Autodesk Inventor part; units mm, degrees
ref_plane "Work Plane2" through (0, 130.175, -69.85) normal (0, 1, 0) x (1, 0, 0)
ref_plane "YZ Plane" through (0, 0, 0) normal (1, 0, 0) x (0, 1, 0)
ref_plane "XZ Plane" through (0, 0, 0) normal (0, 1, 0) x (-1, 0, 0)
ref_plane "Work Plane2" through (0, 130.175, -69.85) normal (0, 1, 0) x (1, 0, 0)
sketch "Sketch3" plane through (0, 130.175, -69.85) normal (0, 1, 0) x (1, 0, 0)
  line L0 (466.5934, -88.9) -> (346.2066, -88.9)
  arc A0 (343.457, -87.3125) -> (346.2066, -88.9) centre (346.2066, -85.725) ccw
  line L1 (334.2915, -71.4375) -> (343.457, -87.3125)
  line L2 (453.2877, 2.1413) -> (445.3167, 25.2907)
  arc A1 (445.3167, 25.2907) -> (442.3147, 27.432) centre (442.3147, 24.257) ccw
  line L3 (370.4853, 27.432) -> (442.3147, 27.432)
  arc A2 (370.4853, 27.432) -> (367.4833, 25.2907) centre (370.4853, 24.257) ccw
  line L4 (367.4833, 25.2907) -> (359.5123, 2.1413)
  arc A3 (356.5103, 0) -> (359.5123, 2.1413) centre (356.5103, 3.175) ccw
  line L5 (355.6, 0) -> (356.5103, 0)
  line L6 (355.6, 0) -> (0, 0)
  line L7 (0, 0) -> (0, -69.85)
  line L8 (0, -69.85) -> (330.2, -69.85)
  line L9 (330.2, -69.85) -> (331.5419, -69.85)
  arc A4 (334.2915, -71.4375) -> (331.5419, -69.85) centre (331.5419, -73.025) ccw
  line L10 (334.2915, -71.4375) -> (343.457, -87.3125)
  arc A5 (343.457, -87.3125) -> (346.2066, -88.9) centre (346.2066, -85.725) ccw
  line L11 (466.5934, -88.9) -> (346.2066, -88.9)
  arc A6 (466.5934, -88.9) -> (469.343, -87.3125) centre (466.5934, -85.725) ccw
  line L12 (469.343, -87.3125) -> (478.5085, -71.4375)
  arc A7 (481.2581, -69.85) -> (478.5085, -71.4375) centre (481.2581, -73.025) ccw
  line L13 (481.2581, -69.85) -> (482.6, -69.85)
  line L14 (482.6, -69.85) -> (812.8, -69.85)
  line L15 (812.8, -69.85) -> (812.8, 0)
  line L16 (812.8, 0) -> (457.2, 0)
  line L17 (456.2897, 0) -> (457.2, 0)
  arc A8 (453.2877, 2.1413) -> (456.2897, 0) centre (456.2897, 3.175) ccw
  circle A9 centre (619.3642, -13.4813) radius 2.667
  circle A10 centre (193.4358, -13.4813) radius 2.667
  circle A11 centre (193.4358, -60.1787) radius 2.667
  arc A12 (666.4551, -57.5409) -> (666.4551, -62.8165) centre (666.0616, -60.1787) ccw
  arc A13 (666.4551, -62.8165) -> (666.4551, -57.5409) centre (666.8486, -60.1787) ccw
  arc A14 (146.3449, -16.1191) -> (146.3449, -10.8435) centre (146.7384, -13.4813) ccw
  arc A15 (146.3449, -10.8435) -> (146.3449, -16.1191) centre (145.9514, -13.4813) ccw
  arc A16 (146.3449, -62.8165) -> (146.3449, -57.5409) centre (146.7384, -60.1787) ccw
  arc A17 (146.3449, -57.5409) -> (146.3449, -62.8165) centre (145.9514, -60.1787) ccw
  arc A18 (666.4551, -10.8435) -> (666.4551, -16.1191) centre (666.0616, -13.4813) ccw
  arc A19 (666.4551, -16.1191) -> (666.4551, -10.8435) centre (666.8486, -13.4813) ccw
  circle A20 centre (170.0871, -36.83) radius 9.525
  circle A21 centre (619.3642, -60.1787) radius 2.667
  circle A22 centre (642.7129, -36.83) radius 9.525
  circle A23 centre (122.6027, -36.83) radius 9.525
  circle A24 centre (99.254, -60.1787) radius 2.667
  circle A25 centre (99.254, -13.4813) radius 2.667
  circle A26 centre (713.546, -13.4813) radius 2.667
  circle A27 centre (713.546, -60.1787) radius 2.667
  circle A28 centre (690.1973, -36.83) radius 9.525
  circle A29 centre (461.9625, -82.7405) radius 3.4036
  circle A30 centre (350.8375, -82.7405) radius 3.4036
  circle A31 centre (711.2, -3.175) radius 1.27
  circle A32 centre (711.2, -66.675) radius 1.27
  circle A33 centre (762, -66.675) radius 1.27
  circle A34 centre (762, -3.175) radius 1.27
  circle A35 centre (50.8, -66.675) radius 1.27
  circle A36 centre (50.8, -3.175) radius 1.27
  circle A37 centre (101.6, -3.175) radius 1.27
  circle A38 centre (101.6, -66.675) radius 1.27
  circle A39 centre (806.45, -30.353) radius 3.3528
  circle A40 centre (6.35, -30.353) radius 3.3528
  circle A41 centre (787.4, -8.128) radius 3.3528
  circle A42 centre (685.8, -8.128) radius 3.3528
  circle A43 centre (584.2, -8.128) radius 3.3528
  circle A44 centre (533.4, -8.128) radius 3.3528
  circle A45 centre (482.6, -8.128) radius 3.3528
  circle A46 centre (25.4, -8.128) radius 3.3528
  circle A47 centre (127, -8.128) radius 3.3528
  circle A48 centre (228.6, -8.128) radius 3.3528
  circle A49 centre (279.4, -8.128) radius 3.3528
  circle A50 centre (330.2, -8.128) radius 3.3528
  circle A51 centre (450.8881, -70.8889) radius 2.032
  circle A52 centre (361.9119, -70.8889) radius 2.032
  circle A53 centre (367.7539, -70.8889) radius 2.54
  circle A54 centre (445.0461, -70.8889) radius 2.54
  circle A55 centre (368.808, 18.0035) radius 2.032
  circle A56 centre (443.992, 18.0035) radius 2.032
  circle A57 centre (374.65, 18.0035) radius 2.54
  circle A58 centre (438.15, 18.0035) radius 2.54
  circle A59 centre (367.6757, 1.016) radius 4.7625
  circle A60 centre (367.6757, -49.784) radius 4.7625
  circle A61 centre (445.1243, -49.784) radius 4.7625
  circle A62 centre (445.1243, 1.016) radius 4.7625
  circle A63 centre (367.6757, -24.384) radius 4.7625
  circle A64 centre (445.1243, -24.384) radius 4.7625
  circle A65 centre (406.4, -11.8872) radius 11.1125
  circle A66 centre (641.35, -55.118) radius 3.3528
  circle A67 centre (546.1, -55.118) radius 3.3528
  circle A68 centre (266.7, -55.118) radius 3.3528
  circle A69 centre (171.45, -55.118) radius 3.3528
  circle A70 centre (513.9255, -52.3027) radius 3.3528
  circle A71 centre (298.8745, -52.3027) radius 3.3528
  circle A72 centre (628.9477, -50.8) radius 4.826
  circle A73 centre (601.4385, -50.8) radius 4.826
  circle A74 centre (568.9249, -50.8) radius 4.826
  circle A75 centre (243.8751, -50.8) radius 4.826
  circle A76 centre (211.3615, -50.8) radius 4.826
  circle A77 centre (183.8523, -50.8) radius 4.826
  circle A78 centre (678.9442, -49.022) radius 4.826
  circle A79 centre (701.4504, -49.022) radius 4.826
  circle A80 centre (726.4609, -49.022) radius 4.826
  circle A81 centre (133.8558, -49.022) radius 4.826
  circle A82 centre (111.3496, -49.022) radius 4.826
  circle A83 centre (86.3391, -49.022) radius 4.826
  circle A84 centre (406.4, -52.578) radius 14.2875
  line L18 (826.5143, 100.4197) -> (706.1275, 100.4197)
  line L19 (813.2086, 191.4611) -> (805.2376, 214.6104)
  arc A85 (805.2376, 214.6104) -> (802.2356, 216.7517) centre (802.2356, 213.5767) ccw
  line L20 (730.4062, 216.7517) -> (802.2356, 216.7517)
  arc A86 (730.4062, 216.7517) -> (727.4042, 214.6104) centre (730.4062, 213.5767) ccw
  line L21 (727.4042, 214.6104) -> (719.4332, 191.4611)
  arc A87 (716.4312, 189.3197) -> (719.4332, 191.4611) centre (716.4312, 192.4947) ccw
  line L22 (715.5209, 189.3197) -> (716.4312, 189.3197)
  line L23 (826.5143, 100.4197) -> (706.1275, 100.4197)
  arc A88 (826.5143, 100.4197) -> (829.2639, 102.0072) centre (826.5143, 103.5947) ccw
  line L24 (816.2106, 189.3197) -> (817.1209, 189.3197)
  arc A89 (813.2086, 191.4611) -> (816.2106, 189.3197) centre (816.2106, 192.4947) ccw
  circle A90 centre (821.8834, 106.5792) radius 3.4036
  circle A91 centre (710.7584, 106.5792) radius 3.4036
  circle A92 centre (810.809, 118.4309) radius 2.032
  circle A93 centre (721.8328, 118.4309) radius 2.032
  circle A94 centre (727.6748, 118.4309) radius 2.54
  circle A95 centre (804.967, 118.4309) radius 2.54
  circle A96 centre (728.7289, 207.3233) radius 2.032
  circle A97 centre (803.9129, 207.3233) radius 2.032
  circle A98 centre (734.5709, 207.3233) radius 2.54
  circle A99 centre (798.0709, 207.3233) radius 2.54
  circle A100 centre (727.5966, 190.3357) radius 4.7625
  circle A101 centre (727.5966, 139.5357) radius 4.7625
  circle A102 centre (805.0452, 139.5357) radius 4.7625
  circle A103 centre (805.0452, 190.3357) radius 4.7625
  circle A104 centre (727.5966, 164.9357) radius 4.7625
  circle A105 centre (805.0452, 164.9357) radius 4.7625
  circle A106 centre (766.3209, 177.4325) radius 11.1125
  circle A107 centre (766.3209, 136.7417) radius 14.2875
  line L25 (817.1209, 189.3197) -> (829.2639, 189.3197)
  line L26 (829.2639, 189.3197) -> (829.2639, 102.0072)
  line L27 (715.5209, 189.3197) -> (706.1275, 189.3197)
  line L28 (706.1275, 100.4197) -> (372.0639, 100.4197)
  line L29 (706.1275, 189.3197) -> (372.0639, 189.3197)
  line L30 (372.0639, 189.3197) -> (372.0639, 100.4197)
  circle A108 centre (-60.9174, 139.5357) radius 4.7625
  circle A109 centre (-60.8392, 118.4309) radius 2.54
  circle A110 centre (-66.6812, 118.4309) radius 2.032
  circle A111 centre (-77.7556, 106.5792) radius 3.4036
  arc A112 (-85.1361, 102.0072) -> (-82.3864, 100.4197) centre (-82.3864, 103.5947) ccw
  circle A113 centre (-60.9174, 164.9357) radius 4.7625
  line L31 (-72.0828, 189.3197) -> (-72.9931, 189.3197)
  arc A114 (-72.0828, 189.3197) -> (-69.0807, 191.4611) centre (-72.0828, 192.4947) ccw
  circle A115 centre (-60.9174, 190.3357) radius 4.7625
  circle A116 centre (-59.7851, 207.3233) radius 2.032
  circle A117 centre (-53.9431, 207.3233) radius 2.54
  arc A118 (16.7237, 214.6104) -> (13.7216, 216.7517) centre (13.7216, 213.5767) ccw
  line L32 (16.7237, 214.6104) -> (24.6946, 191.4611)
  arc A119 (24.6946, 191.4611) -> (27.6966, 189.3197) centre (27.6966, 192.4947) ccw
  line L33 (28.6069, 189.3197) -> (27.6966, 189.3197)
  circle A120 centre (16.5312, 190.3357) radius 4.7625
  circle A121 centre (9.5569, 207.3233) radius 2.54
  circle A122 centre (15.3989, 207.3233) radius 2.032
  line L34 (-82.3864, 100.4197) -> (38.0003, 100.4197)
  circle A123 centre (33.3694, 106.5792) radius 3.4036
  circle A124 centre (22.295, 118.4309) radius 2.032
  circle A125 centre (16.453, 118.4309) radius 2.54
  circle A126 centre (16.5312, 139.5357) radius 4.7625
  circle A127 centre (16.5312, 164.9357) radius 4.7625
  circle A128 centre (-22.1931, 136.7417) radius 14.2875
  circle A129 centre (-22.1931, 177.4325) radius 11.1125
  line L35 (13.7216, 216.7517) -> (-58.1078, 216.7517)
  arc A130 (-58.1078, 216.7517) -> (-61.1098, 214.6104) centre (-58.1078, 213.5767) ccw
  line L36 (-69.0807, 191.4611) -> (-61.1098, 214.6104)
  line L37 (-82.3864, 100.4197) -> (38.0003, 100.4197)
  line L38 (-72.9931, 189.3197) -> (-85.1361, 189.3197)
  line L39 (-85.1361, 189.3197) -> (-85.1361, 102.0072)
  line L40 (28.6069, 189.3197) -> (38.0003, 189.3197)
  line L41 (38.0003, 100.4197) -> (372.0639, 100.4197)
  line L42 (38.0003, 189.3197) -> (372.0639, 189.3197)
  dimension "d7" = 123.1364
  dimension "d8" = 457.2
extrude "Extrusion3" add sketch "Sketch3" along normal blind 3.175 contours L18 L28 L30 L29 L27 L22 A87 L21 A86 L20 A85 L19 A89 L24 L25 L26 A88 | L41 L34 A112 L39 L38 L31 A114 L36 A130 L35 A118 L32 A119 L33 L40 L42 L30
properties part number "am-2952 AM14U2 Inside Sheet Mec Mod"
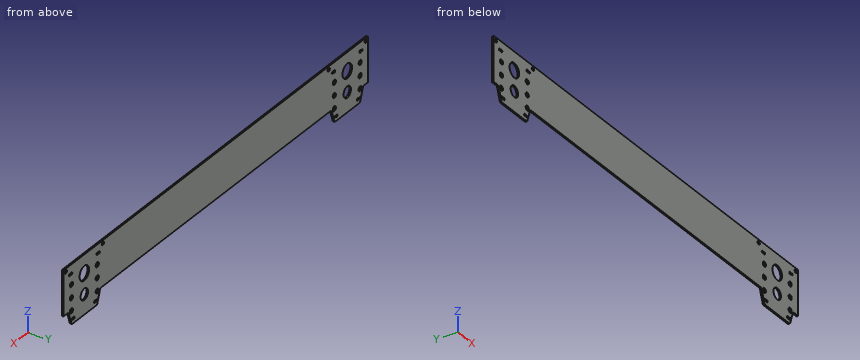
Geometry: final body of the model. Coordinates: model frame, mm. Give positions to 0.01 mm unless a question says otherwise; leave off trailing zeros. Order: outer loops, then holes, each group sorted by start corner. A loop starts at its lowest first (then second) coordinate and runs counter-clockwise, first axis right, second up. Notation, with made-up numbers: (-37.75, 20.5) - (-0.75, 20.5) arc R11 ccw to (-0.75, 25.5) - close; hole circle Ø7 at (-35, 41). An arc over 180 degrees is marked (long way). Use CSV: the item, a comma, the result in double quotes.
1. Section query A-A (x = 601). Output: boundary loops of the cut face in (y, z) (3 decimals).
Answers below:
outline,"(130.175, -259.17) - (133.35, -259.17) - (133.35, -170.27) - (130.175, -170.27) - close"
2. Material intervals for line 1 along X through (y, z) = (133.1, -246); line 2 along Z through (x, y) = (765, 133.05); line 3 along X through (y, z) = (130.9, -235.5), sorted ascending. Write a range as from..to.
Answers below:
line 1,"-85.14..-33.23, -11.15..755.28, 777.36..829.26"
line 2,"-286.6..-258.32, -236.25..-220.82, -192.37..-170.27"
line 3,"-85.14..-65.63, -56.21..11.82, 21.24..722.89, 732.31..800.34, 809.75..829.26"
3. Contact query for flat-ended pins moving along their axis: pin 1 (7.5 mm diameter, centred on x = 727.6, z = -260.19, fed in from -Y); pin 2 (8 mm diameter, centred on x = 33.37, z = -176.43, fed in from -Y) (3 decimals); pin 3 (1 mm diameter, centred on x = -78, y = 132, fed in from -Z). Output: stop coordinate, or through.
Answers below:
pin 1,"through"
pin 2,"y = 130.175"
pin 3,"z = -259.17"
4. Section query B-B (y = 131). Give the number of separate pieces and of enclosed holes in the cut face, plus the area to 3 significant figures.
Answers below:
separate pieces,"1"
enclosed holes,"36"
area,"82,700 mm2"
